Design review of the part built by this model. Coordinates are the model's own, in mm. Give positions to 0.01 mm unless a question says otherwise; leave off trailing zeros. Order: outer loops, then holes, each group sorted by start corner. A loop starts at its lowest first (then second) coordinate and runs counter-clockwise, first axis right, second up.
```python
from build123d import *

# Parameters (mm, degrees)
F0_R     = 13.9065
F0_R_2   = 9.906
F1_DEPTH = 3.175


# Not quite as in the source:
# - a length typed as a fraction of an inch, garbled in the dataset ("3 / 203.2 mm" for 3/8 in), is restored


with BuildPart() as f1:
    # F0 (on Top) → F1 (new body)
    with BuildSketch(Plane.XY):
        with BuildLine():
            Line((-29.0468705796, 64.4645603781), (-113.5004093806, 26.4109228888))
            ThreePointArc((-113.5004093806, 26.4109228888), (-130.5681996552, 0), (-113.5004093806, -26.4109228888))
            Line((-113.5004093806, -26.4109228888), (-29.0468705796, -64.4645603781))
            ThreePointArc((-29.0468705796, -64.4645603781), (70.706437014, 0), (-29.0468705796, 64.4645603781))
        make_face()
        with Locations((-101.6, 0)):
            Circle(F0_R, mode=Mode.SUBTRACT)
        with BuildLine():
            ThreePointArc((0, 64.77), (45.7993062175, 45.7993062175), (64.77, 0))
            ThreePointArc((64.77, 0), (45.7993062175, -45.7993062175), (0, -64.77))
            ThreePointArc((0, -64.77), (-45.7993062175, -45.7993062175), (-64.77, 0))
            ThreePointArc((-64.77, 0), (-45.7993062175, 45.7993062175), (0, 64.77))
        make_face(mode=Mode.SUBTRACT)
        with Locations((-101.6, 0)):
            Circle(F0_R)
        with Locations((-101.6, 0)):
            Circle(F0_R_2, mode=Mode.SUBTRACT)
        with BuildLine():
            Line((0, 9.906), (0, 64.77))
            ThreePointArc((0, 64.77), (-45.7993062175, 45.7993062175), (-64.77, 0))
            Line((-64.77, 0), (-9.906, 0))
            ThreePointArc((-9.906, 0), (-7.0045997744, 7.0045997744), (0, 9.906))
        make_face()
        with BuildLine():
            ThreePointArc((-64.77, 0), (-45.7993062175, -45.7993062175), (0, -64.77))
            Line((0, -64.77), (0, -9.906))
            ThreePointArc((0, -9.906), (-7.0045997744, -7.0045997744), (-9.906, 0))
            Line((-9.906, 0), (-64.77, 0))
        make_face()
        with BuildLine():
            ThreePointArc((0, -64.77), (45.7993062175, -45.7993062175), (64.77, 0))
            ThreePointArc((64.77, 0), (45.7993062175, 45.7993062175), (0, 64.77))
            Line((0, 64.77), (0, 9.906))
            ThreePointArc((0, 9.906), (7.0045997744, 7.0045997744), (9.906, 0))
            ThreePointArc((9.906, 0), (7.0045997744, -7.0045997744), (0, -9.906))
            Line((0, -9.906), (0, -64.77))
        make_face()
    extrude(amount=F1_DEPTH)


solid = f1.part
```
1. Take a section at A-A (z = 2.35). State the section outline as (x, y) points, then the cut area to 3 significant figures.
Recorded:
outline: (-113.5, -26.41) - (-29.05, -64.46) arc R70.71 ccw (long way) to (-29.05, 64.46) - (-113.5, 26.41) arc R28.97 ccw to start; hole circle Ø19.81 at (-101.6, 0); hole circle Ø19.81 at (0, 0)
area: 19,500 mm2
2. Take a section at D-D (y = -55.5). State the section outline as (x, z) points (3 decimals).
Recorded:
outline: (-48.942, 0) - (43.808, 0) - (43.808, 3.175) - (-48.942, 3.175) - close
3. For pin 1 (1.5 mm diameter, centred on x = -65, z = 1.5, fed in from -Y); pin 2 (1.5 mm diameter, centred on x = -100.5, z = 2, fed in from +Y); pin 3 (1 mm diameter, centred on y = 54.5, z = 2.5, fed in from +X); pin 4 (18 mm diameter, centred on x = -101.6, y = 0, fed in from +Z), all flat-tipped, find the tip position at first contact; note any pin that passes through.
Recorded:
pin 1: stops at y = -48.6
pin 2: stops at y = 32.61
pin 3: stops at x = 45.64
pin 4: passes through
4. Take a section at C-C (x = 4). State the section outline as (y, z) points (1 decimal), then the cut area to 3 significant figures.
Recorded:
outline: (-70.6, 0) - (-9.1, 0) - (-9.1, 3.2) - (-70.6, 3.2) - close; (9.1, 0) - (70.6, 0) - (70.6, 3.2) - (9.1, 3.2) - close
area: 391 mm2
5. Draft analysis for pull direction X (two halves, no side actions). For faces 1 (the face through (-31, 1, 0)), 2 (the face through (-108.901, 6.695, 1.565)), 3 (the face through (70.68, -1.97, 1.57)), 4 (the face through (-70.682, 45.704, 1.565)), state which applies: pulls with the +X half, pulls with the -X half, needs draft (parallel to the pull), parting line crosses it, or undercut.
Recorded:
face 1: needs draft
face 2: undercut
face 3: parting line crosses it
face 4: pulls with the -X half
6. Take a section at B-B (x = -101.6). State the section outline as (y, z) points (3 decimals), then the cut area to 3 significant figures.
Recorded:
outline: (-31.773, 0) - (-9.906, 0) - (-9.906, 3.175) - (-31.773, 3.175) - close; (9.906, 0) - (31.773, 0) - (31.773, 3.175) - (9.906, 3.175) - close
area: 139 mm2
7. For line 1 along X through (y, z) = (-9, 1.55); line 2 along X through (y, z) = (-1, 0.75); line 3 along Y through (x, z) = (-101.6, 2.15), list the stretches that pass through material, from the lowest coordinate up.
Recorded:
line 1: x = -129.13 to -105.74, -97.46 to -4.14, 4.14 to 70.13
line 2: x = -130.55 to -111.46, -91.74 to -9.86, 9.86 to 70.7
line 3: y = -31.77 to -9.91, 9.91 to 31.77
